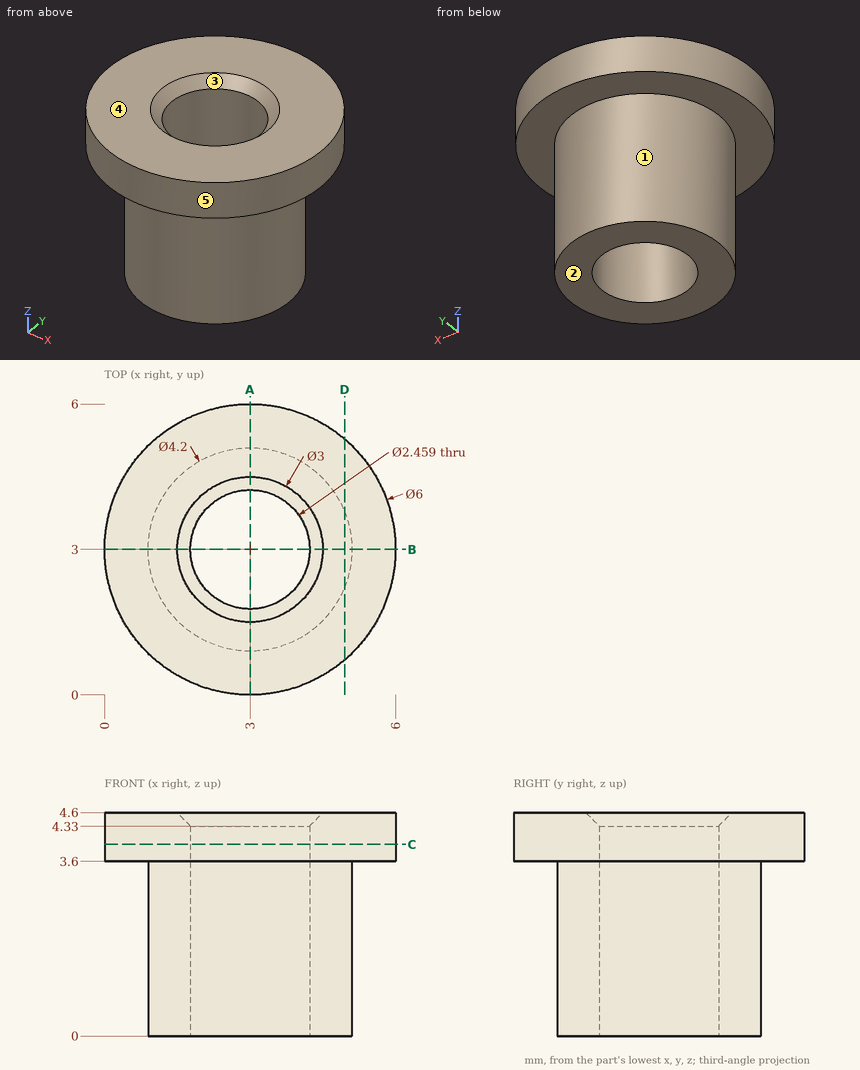
For this review, use the dimensioned drawing (mm, ordinates from the lowest corner) and the shaded views. A direction names the side the tool comes from. Give positions to 0.01 mm unless a question says otherwise; leave off trailing zeros. Loops run counter-clockwise (first coordinate to the right, second up) from the corner with the lowest first, then second, coordinate; pieces in that order, holes last.
Item 1: For line 1 along Y through (x, z) = (3, 1.95); line 2 along Z through (x, y) = (1.05, 1.15), list the stretches that pass through material, from the lowest coordinate up.
Item 2: Draft analysis for pull direction Y (two halves, no side actions). For the marked faces 3, 4 and 5, state which applies: +Y half, -Y half, draft (parallel to the pull), parting line (faces both ways), or undercut.
Item 3: Tool access review of the marked faces 1 and 2: name each direction out of +Z, -Z, +X, -X, +Y, -Y from which nothing blocks a thin tool from reaching the whole face with its end or side.
Item 4: Take a section at A-A, the plane x = 3. State the section outline as (y, z) points.
Item 5: Take a section at C-C, the plane z = 3.95. State the section outline as (x, y) points.
Item 6: Insertion check: pin 1 (2 mm diameter, centred on x = 1, z = 3.5, fed in from +Y); pin 2 (1.5 mm diameter, centred on x = 5.5, y = 1.5, fed in from -Z); pin 3 (1.5 mm diameter, centred on x = 2, z = 3, fed in from +Y). Each pin has a flat end and moves straight along its axis. Give the tip position at first contact, or say it passes through.
Item 7: Take a section at D-D, the plane x = 4.95. State the section outline as (y, z) points, and give its area (3 significant figures).
Calculated:
1. line 1: y = 0.9 to 1.77, 4.23 to 5.1
1. line 2: z = 3.6 to 4.6
2. face 3: undercut
2. face 4: draft
2. face 5: parting line
3. face 1: -Z
3. face 2: -Z, +X, -X, +Y, -Y
4. outline: (0, 3.6) - (0.9, 3.6) - (0.9, 0) - (1.77, 0) - (1.77, 4.33) - (1.5, 4.6) - (0, 4.6) - close; (4.23, 0) - (5.1, 0) - (5.1, 3.6) - (6, 3.6) - (6, 4.6) - (4.5, 4.6) - (4.23, 4.33) - close
5. outline: circle Ø6 at (3, 3); hole circle Ø2.46 at (3, 3)
6. pin 1: stops at y = 5.83
6. pin 2: stops at z = 3.6
6. pin 3: stops at y = 5.95
7. outline: (0.72, 3.6) - (2.22, 3.6) - (2.22, 0) - (3.78, 0) - (3.78, 3.6) - (5.28, 3.6) - (5.28, 4.6) - (0.72, 4.6) - close
7. area: 10.2 mm2
